The figure shows three views and two pictorial views of one solid part (mm, origin at its lowest corner). Answer the questions. A direction names the side the tool comes from. Round coordinates to 2 decimals unless told otherwise and drop trailing zeros. Order: outer loops, then holes, each group sorted by start corner. A loop starts at its lowest first (then second) coordinate and runs counter-clockwise, first axis right, second up. Notation, with made-up numbers: (60, 10) - (102, 10) arc R21 cw to (102, 20) - close; hole circle Ø1 at (12, 12). An arc over 180 degrees is marked (long way). Write item = value, one per line.
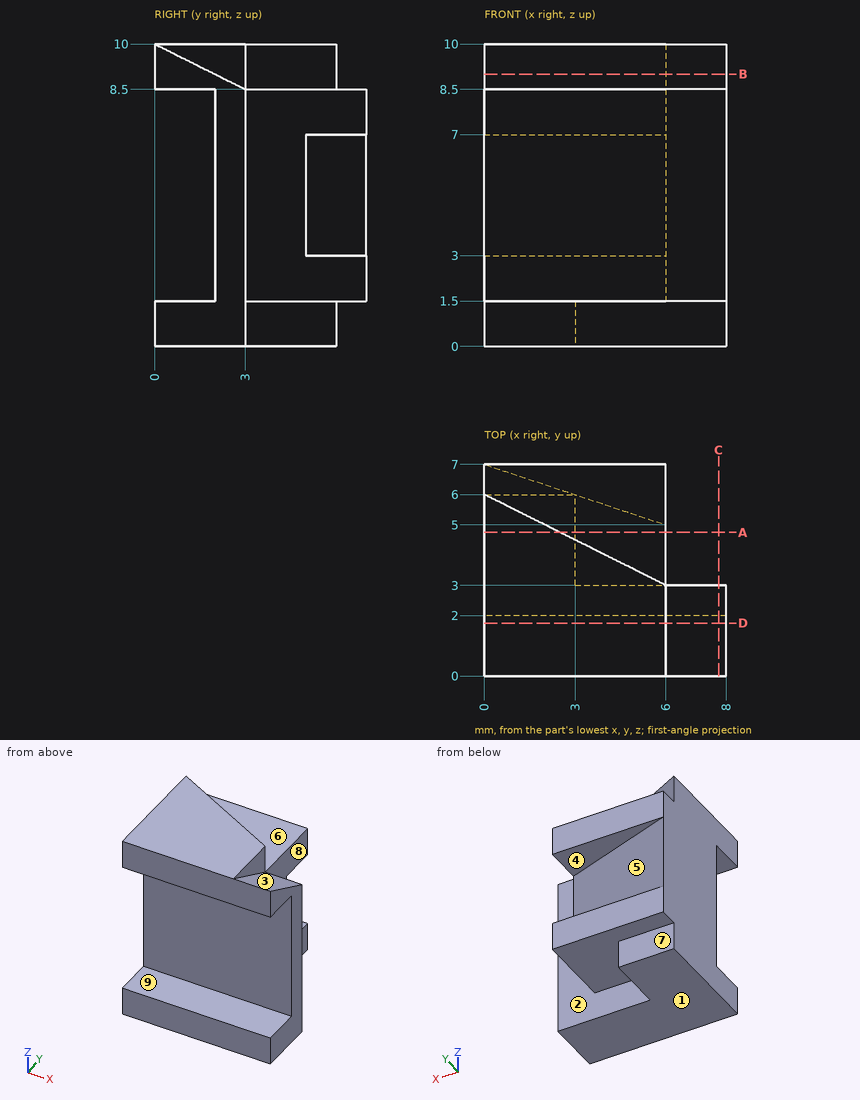
Q1. Flat-ended cylindrical pins translate along their axes: P1, Ø1.2, axis at y = 5.5, z = 4.5, coming from the +X side; P2, Ø1.2, axis at x = 4, y = 5, coming from the +Z side; P3, Ø1, axis at x = 4.5, y = 5.5, coming from the -Z side. Find the tip coordinate at first contact, or state that the pin passes through.
Model answer:
P1 = 6
P2 = 8.5
P3 = 1.5
Q2. Section A-A on y = 4.75 is taken. Determine the outline of the cut face in (x, z), then the cut area to 4 significant figures.
Model answer:
outline = (0, 0) - (3, 0) - (3, 1.5) - (6, 1.5) - (6, 8.5) - (2.5, 8.5) - (2.5, 10) - (0, 10) - close
area = 50.25 mm^2
Q3. Section D-D on y = 1.75 is taken. Determine the outline of the cut face in (x, z) (3 decimals), then the cut area to 4 significant figures.
Model answer:
outline = (0, 0) - (8, 0) - (8, 1.5) - (0, 1.5) - close; (0, 8.5) - (8, 8.5) - (8, 9.125) - (6, 9.125) - (6, 10) - (0, 10) - close
area = 22.25 mm^2
Q4. Determine the mould class of the marked faces 1, 2, 3 and 4 for opening direction Z: released by +Z, released by -Z, zero draft, split by the parting line, or undercut.
Model answer:
face_1 = released by -Z
face_2 = zero draft
face_3 = released by +Z
face_4 = undercut
Q5. Section B-B on z = 9 is taken. Determine the outline of the cut face in (x, y).
Model answer:
outline = (0, 0) - (8, 0) - (8, 2) - (6, 2) - (6, 3) - (0, 6) - close
Q6. Section C-C on x = 7.75 is taken. Determine the outline of the cut face in (y, z), then the cut area to 4 significant figures.
Model answer:
outline = (0, 0) - (3, 0) - (3, 8.5) - (0, 10) - (0, 8.5) - (2, 8.5) - (2, 1.5) - (0, 1.5) - close
area = 13.75 mm^2
Q7. For the marked faces 5, 6, 7, 8 and 9, determine the directions among +Z, -Z, +X, -X, +Y, -Y from which every point of the face is accessible in a straight line to the end or side of a thin tool.
Model answer:
face_5 = +X, +Y
face_6 = +Z, +X, +Y
face_7 = -Z, +X, -X, +Y
face_8 = +Z, -Z, +X, +Y
face_9 = +X, -X, -Y
Q8. Find the intervals of material crossed by line 1 (Z direction, x = 4, y = 0.5); line 2 (Z direction, x = 5.25, y = 5); line 3 (Y direction, x = 5.25, z = 1), in increasing order. Write a range as from..to.
Model answer:
line_1 = 0..1.5, 8.5..10
line_2 = 1.5..8.5
line_3 = 0..3
